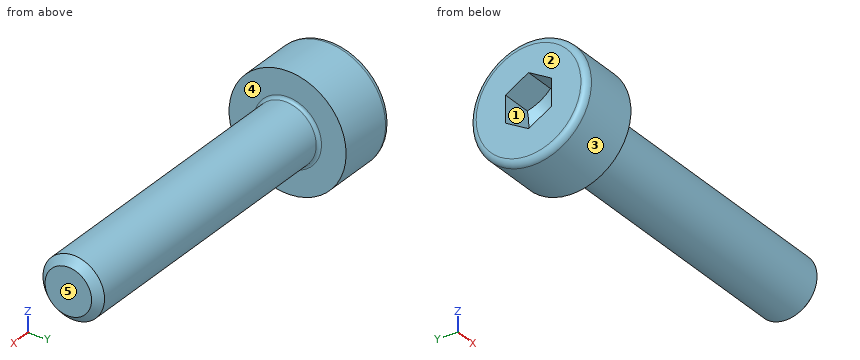
Autodesk Inventor part; units mm, degrees
ref_plane "Work Plane1" through (29, 0, 0) normal (0, -1, 0) x (1, 0, 0)
ref_plane "YZ Plane" through (0, 0, 0) normal (1, 0, 0) x (0, 1, 0)
ref_plane "XZ Plane" through (0, 0, 0) normal (0, 1, 0) x (-1, 0, 0)
sketch "Skizze1" plane through (0, 0, 0) normal (0, 0, 1) x (1, 0, 0)
  line L0 (-0.5, 0) -> (10, 0)
  line L1 (10, 0) -> (10, 1)
  line L2 (10, 1) -> (1.2, 1)
  line L3 (1.2, 1) -> (0.9545, 1)
  line L4 (0.9545, 1) -> (0, 1)
  line L5 (0, 1) -> (0, 1.9)
  line L6 (0, 1.9) -> (-2, 1.9)
  line L7 (-2, 1.9) -> (-2, 0.866)
  line L8 (-2, 0.866) -> (-1, 0.866)
  line L9 (-1, 0.866) -> (-0.5, 0)
  line L10 (-4.4, 0) -> (12.4, 0)
  line L11 (0, -0.38) -> (0, 2.28)
  line L12 (1.2, 1) -> (0, 1) construction
  dimension "d1" = 8.8
  dimension "d2" = 0.2455
  dimension "d3" = 2
  dimension "d4" = 1
  dimension "d5" = 60
  dimension "d6" = 2
  dimension "d7" = 2
  dimension "d8" = 1.7321
  dimension "d9" = 3.8
  dimension "d26" = 10
revolve "Körper" add sketch "Skizze1" angle 360 about axis through (-0.5, 0, 0) along (1, 0, 0)
sketch "Skizze2" plane through (-2, 0, 0) normal (-1, 0, 0) x (0, 0, 1)
  circle A0 centre (0, 0) radius 0.866
  line L0 (0, -2.66) -> (0, 2.66)
  line L1 (-2.66, 0) -> (2.66, 0)
  line L2 (0.866, 0) -> (0.433, -0.75)
  line L3 (0.433, -0.75) -> (-0.433, -0.75)
  line L4 (-0.433, -0.75) -> (-0.866, 0)
  line L5 (-0.866, 0) -> (-0.433, 0.75)
  line L6 (-0.433, 0.75) -> (0.433, 0.75)
  line L7 (0.433, 0.75) -> (0.866, 0)
  point P0 (0, 0)
extrude "Loch" add sketch "Skizze2" against normal up to next contours L7 A0 | A0 L2 | L6 L0 A0 | A0 L0 L3 | L0 L6 A0 | A0 L3 L0 | L4 A0 | A0 L5
fillet "Rundung1" radius 0.2 1 edges at (-2, -1.9, 0)
thread "Gewinde"
chamfer "Fase1" distance 0.2454 distance2 0.2454 1 edges at (10, -1, 0) measured on face at (10, -0.5392, -0.3309)
ref_plane "Work Plane1" through (29, 0, 0) normal (0, -1, 0) x (1, 0, 0)
fillet "Fillet2" radius 0.1 1 edges at (0, -1, 0)
equation "\"d1\" = GEL"
equation "\"d3\" = KOH"
equation "\"d4\" = INTI"
equation "\"d6\" = GD"
equation "\"d7\" = BDM"
equation "\"d8\" = 1.1547 * SW"
equation "\"d9\" = KOD"
equation "\"d26\" = NLG"
equation "\"d30\" = R"
equation "\"d17\" = RR"
equation "\"d13\" = GEL"
equation "\"d15\" = -0.5 * SPD + 0.5 * GD"
equation "\"d16\" = GUL"
equation "\"GD\" = 2"
equation "\"NLG\" = 10"
equation "\"GEL\" = 8.8"
equation "\"KOD\" = 3.8"
equation "\"KOH\" = 2"
equation "\"INTI\" = 1"
equation "\"GAL\" = 0.61345 * PTC"
equation "\"GUL\" = 0.61345 * PTC"
equation "\"BDM\" = NND"
equation "\"SW\" = 1.5"
equation "\"RR\" = 0.2"
equation "\"SPD\" = NND - 1.2269 * PTC"
equation "\"R\" = 0.1"
equation "\"TOA\" = 30deg"
equation "\"GD1\" = THREADDIA - 1.2269 * PTC"
equation "\"THREADDIA\" = 2"
equation "\"FAWI\" = 45deg"
equation "\"PTC\" = 0.4"
equation "\"NND\" = 2"
equation "\"E0\" = 1.155 * SW"
properties part number "ISO 4762  - M2 x 10" material "Edelstahl, 440C"
Could you check a few things on this model? Use its own coordinates, in mm. Face numbers are marked on the shaded views. A direction names the side the tool comes from. Round coordinates to 2 decimals unless told otherwise and drop trailing zeros. Write each loop counter-clockwise with the first axis right and the second up, starting at its lowest first coordinate (ties: lowest second). Pieces come first, ordered by that corner, then holes. Notation, with made-up numbers: (72.25, 12.5) - (107.25, 12.5) arc R13 cw to (107.25, 36.5) - close; hole circle Ø3 at (-18, -26.5). An arc over 180 degrees is marked (long way). Use a Markdown table: item, result.
Q1. For the marked faces 4 and 5, which set-ups out of +Z, -Z, +X, -X, +Y, -Y let a thin tool reach every point of the face, with its end or its side?
Output values:
| item | result |
|---|---|
| face 4 | +X |
| face 5 | +Z, -Z, +X, +Y, -Y |
Q2. For pin 1 (1 mm diameter, centred on x = 1, y = 0.5, fed in from +Z); pin 2 (1.5 mm diameter, centred on x = 7, z = 1.5, fed in from +Y), each with a flat end and sliding along its axis, tell me the tip position at first contact or that it passes through.
Output values:
| item | result |
|---|---|
| pin 1 | z = 1 |
| pin 2 | y = 0.66 |
Q3. Please list where these lines run through material, in increasing order: L1, parallel to X at y = -0.35, z = 1.05; L2, parallel to Y at x = 5, z = 0.9; L3, parallel to Z at x = 4.75, y = -0.5.
Output values:
| item | result |
|---|---|
| L1 | -2 to 0 |
| L2 | -0.44 to 0.44 |
| L3 | -0.87 to 0.87 |
Q4. Thinking about a two-plate mould opening in Y: for the marked faces 1, 2 and 3, which applies, released by +Y, released by -Y, zero draft, split by the parting line, or undercut?
Output values:
| item | result |
|---|---|
| face 1 | undercut |
| face 2 | zero draft |
| face 3 | split by the parting line |
Q5. I want a section at B-B (x = 6.5). List the corners of the cut face in (y, z) for me, plus the area to 3 significant figures.
Output values:
| item | result |
|---|---|
| outline | circle Ø2 at (0, 0) |
| area | 3.14 mm2 |
Q6. I want a section at A-A (x = -0.25). List the corners of the cut face in (y, z) for me.
Output values:
| item | result |
|---|---|
| outline | circle Ø3.8 at (0, 0) |
